Solid Edge part; units mm, degrees
sketch "Sketch1" plane through (0, 0, 0) normal (0, -1, 0) x (1, 0, 0)
  line L0 (-47, -47) -> (47, -47)
  line L1 (47, -47) -> (47, 47)
  line L2 (47, 47) -> (-47, 47)
  line L3 (-47, 47) -> (-47, -47)
extrude "Protrusion1" add sketch "Sketch1" against normal blind 0.2
sketch "Sketch2" plane through (0, 0.2, 0) normal (0, 1, 0) x (0, 0, -1)
  line L0 (-31.0077, 45.5) -> (-31.0077, 33.4066)
  line L1 (-31.0077, 33.4066) -> (-46, 33.4066)
  line L2 (-46, 33.4066) -> (-46, -38.6606)
  line L3 (-46, -38.6606) -> (-35.6145, -38.6606)
  line L4 (-35.6145, -38.6606) -> (-35.6145, -45.5)
  line L5 (-35.6145, -45.5) -> (33.5653, -45.5)
  line L6 (33.5653, -45.5) -> (33.5653, -38.5694)
  line L7 (33.5653, -38.5694) -> (46, -38.5694)
  line L8 (46, -38.5694) -> (46, 34.0082)
  line L9 (46, 34.0082) -> (30.5923, 34.0082)
  line L10 (30.5923, 34.0082) -> (30.5923, 44.4526)
  line L11 (30.5923, 45.5) -> (30.5923, 44.4526)
  line L12 (-31.0077, 45.5) -> (30.5923, 45.5)
  dimension "D1" = 31.0077
  dimension "D2" = 46
  dimension "D3" = 35.6145
  dimension "D4" = 33.5653
  dimension "D5" = 46
extrude "Cutout1" cut sketch "Sketch2" along normal mid plane 166.709 flip side to cut
sketch "Sketch3" plane through (0, 0, 0) normal (0, -1, 0) x (0, 0, 1)
  circle A0 centre (28, 0) radius 1.25
extrude "ExtrudedCutout_4" cut sketch "Sketch3" along normal mid plane 10.5197
sketch "Sketch4" plane through (0, 0, 0) normal (0, -1, 0) x (0, 0, 1)
  circle A0 centre (-28, 0) radius 1.25
extrude "ExtrudedCutout_5" cut sketch "Sketch4" along normal mid plane 893.0188
properties material "Copper"
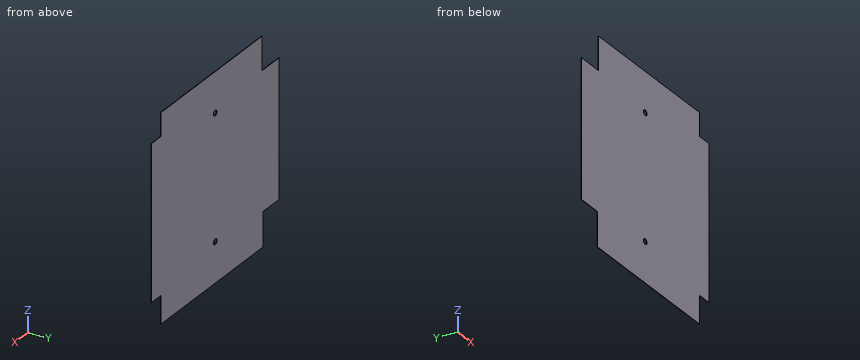
The listing builds one solid part. Answer for the finished solid, in the listing's coordinates (mm). Coordinates: 2 decimals unless noted, no trailing zeros. Write each loop counter-clockwise with the first axis right and the second up, starting at its lowest first coordinate (ties: lowest second). Pieces come first, ordered by that corner, then holes. Notation, with made-up numbers: M 44.25,-11.75 L 53.25,-11.75 A20 cw 53.25,9.25 Z; hole C -1.75,-16.5 d11. An arc over 180 degrees is marked long. Put each result on its own line as item: value. Start each with the question number.
1. A cutting plane is placed at A-A on x = 0. Write down the section's boundary in (y, z).
2. Consider line 1 (Z direction, x = 0, y = 0.15); line 2 (X direction, y = 0.1, z = -28); line 3 (Z direction, x = -0.5, y = 0.05). Determine where each line is inside the solid, lowest interval first. Write a range as from..to.
3. A cutting plane is placed at B-B on z = 28. Write down the section's boundary in (x, y), then the cut area to 3 significant figures.
4. A flat-ended cylindrical pin translates along its axis: P1, Ø1.5, axis at x = 0, z = 28, coming from the +Y side. Find the tip coordinate at first contact, or state that the pin passes through.
5. A cutting plane is placed at C-C on y = 0.15. Write down the section's boundary in (x, z), then the cut area to 3 significant figures.
Resolved:
1. outline: M 0,-46 L 0.2,-46 L 0.2,-29.25 L 0,-29.25 Z; M 0,-26.75 L 0.2,-26.75 L 0.2,26.75 L 0,26.75 Z; M 0,29.25 L 0.2,29.25 L 0.2,46 L 0,46 Z
2. line 1: z = -46..-29.25, -26.75..26.75, 29.25..46
2. line 2: x = -45.5..-1.25, 1.25..45.5
2. line 3: z = -46..-29.15, -26.85..26.85, 29.15..46
3. outline: M -45.5,0 L -1.25,0 L -1.25,0.2 L -45.5,0.2 Z; M 1.25,0 L 45.5,0 L 45.5,0.2 L 1.25,0.2 Z
3. area: 17.7 mm2
4. P1: passes through
5. outline: M -45.5,-30.59 L -34.01,-30.59 L -34.01,-46 L 38.57,-46 L 38.57,-33.57 L 45.5,-33.57 L 45.5,35.61 L 38.66,35.61 L 38.66,46 L -33.41,46 L -33.41,31.01 L -45.5,31.01 Z; hole C 0,-28 d2.5; hole C 0,28 d2.5
5. area: 7,850 mm2
